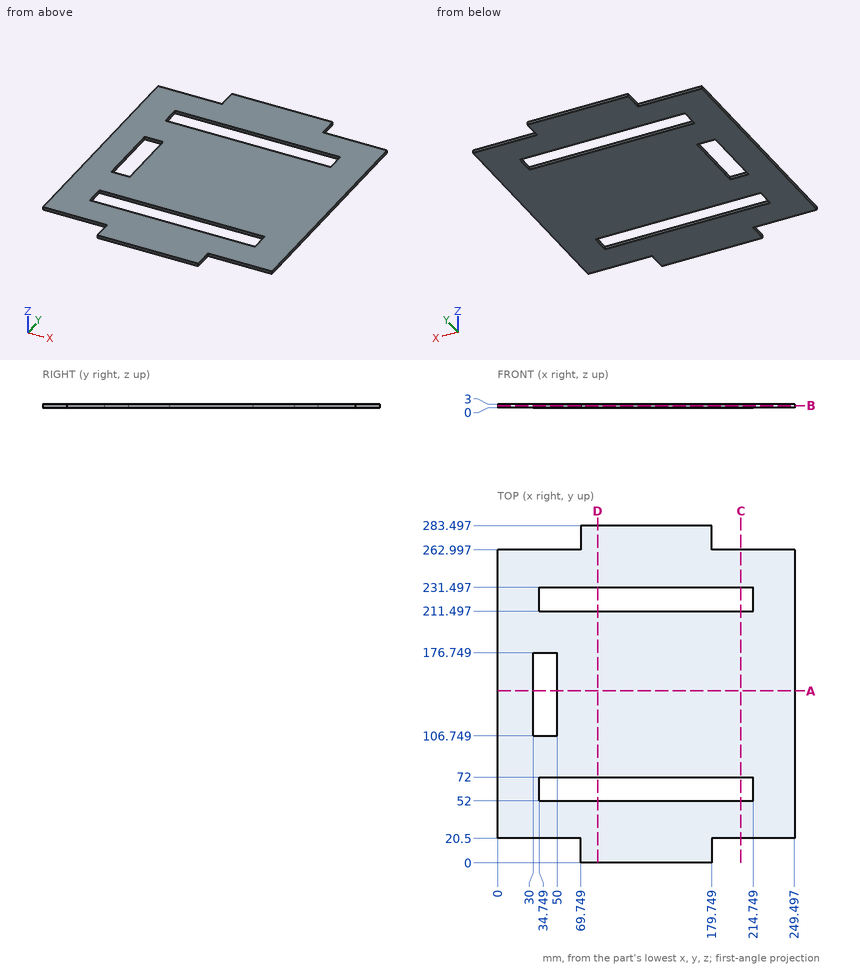
Print and shaded views of the part. All mm, measured from the part's lowest x, y and z. Give positions to 0.01 mm unless a question says otherwise; leave off trailing zeros. Loops run counter-clockwise (first coordinate to the right, second up) from the corner with the lowest first, then second, coordinate; pieces in that order, holes last. Notation, with made-up numbers: (32, 67.5) -> (75, 67.5) arc R14 cw to (75, 90.5) -> close; hole circle Ø11 at (77.25, 5.25). An arc over 180 degrees is marked (long way). Use a Markdown table: item, result.
1. Slice it at D-D (x = 84). List the corners of the cut face in (y, z).
Check result:
| item | result |
|---|---|
| outline | (0, 0) -> (52, 0) -> (52, 3) -> (0, 3) -> close; (72, 0) -> (211.5, 0) -> (211.5, 3) -> (72, 3) -> close; (231.5, 0) -> (283.5, 0) -> (283.5, 3) -> (231.5, 3) -> close |
2. Slice it at A-A (y = 144.5). List the corners of the cut face in (x, z).
Check result:
| item | result |
|---|---|
| outline | (0, 0) -> (30, 0) -> (30, 3) -> (0, 3) -> close; (50, 0) -> (249.5, 0) -> (249.5, 3) -> (50, 3) -> close |
3. Slice it at C-C (x = 204.5). List the corners of the cut face in (y, z).
Check result:
| item | result |
|---|---|
| outline | (20.5, 0) -> (52, 0) -> (52, 3) -> (20.5, 3) -> close; (72, 0) -> (211.5, 0) -> (211.5, 3) -> (72, 3) -> close; (231.5, 0) -> (263, 0) -> (263, 3) -> (231.5, 3) -> close |
4. Flat gauge pins, fed straight in: pin 1 (1 mm diameter, centred on x = 153, y = 189.5, fed in from -Z); pin 2 (0.9 mm diameter, centred on y = 275.5, z = 1.5, fed in from -X); pin 3 (0.9 mm diameter, centred on x = 24, z = 2, fed in from +Y); pin 4 (0.9 mm diameter, centred on x = 220, z = 1, fed in from -Y). Where does each tip first touch, or does it go through?
Check result:
| item | result |
|---|---|
| pin 1 | stops at z = 0 |
| pin 2 | stops at x = 69.75 |
| pin 3 | stops at y = 263 |
| pin 4 | stops at y = 20.5 |
5. Wall check: L1, parallel to Y at x = 184, z = 1.2; L2, parallel to Y at x = 126.5, z = 2.1; L3, parallel to Y at x = 48, z = 1.75. Give the ranges that are in metal, low to high. Write a range as [from, to].
Check result:
| item | result |
|---|---|
| L1 | y = [20.5, 52], [72, 211.5], [231.5, 263] |
| L2 | y = [0, 52], [72, 211.5], [231.5, 283.5] |
| L3 | y = [20.5, 52], [72, 106.75], [176.75, 211.5], [231.5, 263] |
6. Slice it at B-B (z = 1.55). List the corners of the cut face in (x, y).
Check result:
| item | result |
|---|---|
| outline | (0, 20.5) -> (69.75, 20.5) -> (69.75, 0) -> (179.75, 0) -> (179.75, 20.5) -> (249.5, 20.5) -> (249.5, 263) -> (179.75, 263) -> (179.75, 283.5) -> (69.75, 283.5) -> (69.75, 263) -> (0, 263) -> close; hole (30, 106.75) -> (50, 106.75) -> (50, 176.75) -> (30, 176.75) -> close; hole (34.75, 52) -> (214.75, 52) -> (214.75, 72) -> (34.75, 72) -> close; hole (34.75, 211.5) -> (214.75, 211.5) -> (214.75, 231.5) -> (34.75, 231.5) -> close |
